from build123d import *

# Parameters (mm, degrees)
SKETCH1_W           = 5.5
SKETCH1_H           = 2.45
BOSS_EXTRUDE1_DEPTH = 60
BOSS_EXTRUDE2_DEPTH = 60


with BuildPart() as part:
    # Sketch1 → Boss-Extrude1 (new body)
    with BuildSketch(Plane.XY):
        with Locations((0, 1.225)):
            Rectangle(SKETCH1_W, SKETCH1_H)
    extrude(amount=BOSS_EXTRUDE1_DEPTH)

    # Sketch2 → Boss-Extrude2 (add)
    with BuildSketch(Plane.XY):
        Polygon((-4.6, 2.45), (4.6, 2.45), (4.6, 3.085), (2.794, 5.8), (-2.794, 5.8), (-4.6, 3.085), align=None)
    extrude(amount=BOSS_EXTRUDE2_DEPTH)


solid = part.part
Can you work these out from the model? Positions are in its coordinate system, mm. A direction names the side the tool comes from. Coordinates: 2 decimals unless noted, no trailing zeros. Write each loop counter-clockwise with the first axis right and the second up, starting at its lowest first coordinate (ties: lowest second). Pieces come first, ordered by that corner, then holes. Notation, with made-up numbers: (83.5, -28) -> (105.5, -28) arc R17 ccw to (105.5, -4) -> close; hole circle Ø6 at (21, 5). An arc over 180 degrees is marked (long way). Answer as CSV lines item,"result".
1) If we section it at A-A on z = 27: Please give me the cut outline in (x, y) (3 decimals).
Check result:
outline,"(-4.6, 2.45) -> (-2.75, 2.45) -> (-2.75, 0) -> (2.75, 0) -> (2.75, 2.45) -> (4.6, 2.45) -> (4.6, 3.085) -> (2.794, 5.8) -> (-2.794, 5.8) -> (-4.6, 3.085) -> close"
2) If we section it at C-C on x = -3.75: Please give me the cut outline in (y, z), then the cut area to 3 significant figures.
Check result:
outline,"(2.45, 0) -> (4.36, 0) -> (4.36, 60) -> (2.45, 60) -> close"
area,"115 mm²"
3) If I drill on line 1 (X direction, y = 1.35, z = 22); line 2 (X direction, y = 3.35, z = 35.5); line 3 (Y direction, x = 3, z = 8.5), over which ranges is the centre line in solid material (lowest first)? Write a range as from..to.
Check result:
line 1,"-2.75..2.75"
line 2,"-4.42..4.42"
line 3,"2.45..5.49"
4) If we section it at B-B on y = 0.8: Please give me the cut outline in (x, z).
Check result:
outline,"(-2.75, 0) -> (2.75, 0) -> (2.75, 60) -> (-2.75, 60) -> close"
5) Will these pins go through, and if not, where does the flat tip stop? P1, Ø3, axis at x = -3, y = 4.5, coming from the -Z side; P2, Ø2.5, axis at y = 0.5, z = 33.5, coming from the +X side; P3, Ø0.9, axis at x = 4, z = 19.5, coming from the -Y side; P4, Ø2, axis at y = 1, z = 42.5, coming from the -X side.
Check result:
P1,"z = 0"
P2,"x = 2.75"
P3,"y = 2.45"
P4,"x = -2.75"
6) On a 3-axis mill with a long thin cutter (end or side, diameter ignored), from which of +Z, -Z, +X, -X, +Y, -Y can I reach the whole of each face in a straight line? I mean faces 1 (the flat face through (0, 5.8, 30)), 2 (the flat face through (-2.75, 1, 30)), 3 (the flat face through (2.75, 1, 30)). Say none if no direction works.
Check result:
face 1,"+Z, -Z, +X, -X, +Y"
face 2,"+Z, -Z, -X, -Y"
face 3,"+Z, -Z, +X, -Y"
